Part model, mm, in its own coordinate system. A direction names the side the tool comes from. Round coordinates to 2 decimals unless told otherwise and drop trailing zeros. Use a Markdown table: item, result. Add a question column.
Item 1: Which spindle directions (+Z, -Z, +X, -X, +Y, -Y) get a long thin tool onto all of the face, cutting with end or side? Do faces 1 (the face through (-24.724, 24.297, 1.504)), 2 (the face through (1.1, 27.994, 1.504)), 3 (the face through (1.1, 27.994, 8.496)). Say none if no direction does.
Item 2: Flat gauge pins, fed straight in: pin 1 (12 mm diameter, centred on x = -22.5, y = 18.5, fed in from +Z); pin 2 (1.5 mm diameter, centred on x = -11, z = 1.5, fed in from +Y); pin 3 (1 mm diameter, centred on x = -5.5, z = 9, fed in from -Y); pin 4 (5 mm diameter, centred on x = 0.5, y = 28, fed in from -Z). Where does each tip first touch, or does it go through?
Item 3: Probe line 1 (Y direction, x = -24.5, z = 5); line 2 (X direction, y = 28.25, z = 4.75); line 3 (X direction, y = 31.75, z = 3). List the from-to ranges inside material, lowest first. Write a range as [from, to].
```python
from build123d import *

# Parameters (mm, degrees)
F0_W     = 12
F0_H     = 12
F0_W_2   = 10
F0_H_2   = 10
F1_DEPTH = 10
F2_R     = 4.99999


# Not quite as in the source:
# - a fillet or chamfer is up to 0.001 mm smaller than in the source, because OpenCascade refuses the exact size


with BuildPart() as f1:
    # F0 (on Top) → F1 (new body)
    with BuildSketch(Plane.XY):
        Polygon((2.5256457627, 38.7224316552), (-22.4743542373, 38.7224316552), (-22.4743542373, 25.7224316552), (-22.4743542373, 13.7224316552), (2.5256457627, 13.7224316552), (2.5256457627, 23.7224316552), align=None)
        with Locations((-28.4743542373, 19.7224316552)):
            Rectangle(F0_W, F0_H)
        with Locations((7.5256457627, 18.7224316552)):
            Rectangle(F0_W_2, F0_H_2)
    extrude(amount=F1_DEPTH)

    # F2 (radius 5 in the source; OpenCascade refuses exactly that, so slightly less here)
    f2_edges = [f1.edges().sort_by_distance(p)[0] for p in [
        (-22.474354, 38.722432, 5),
        (-22.474354, 32.222432, 10),
        (-34.474354, 19.722432, 10),
        (-34.474354, 25.722432, 5),
        (-34.474354, 13.722432, 5),
        (-34.474354, 19.722432, 0),
        (2.525646, 31.222432, 10),
        (-9.974354, 38.722432, 10),
        (-28.474354, 25.722432, 10),
        (-10.974354, 13.722432, 10),
        (12.525646, 18.722432, 10),
        (7.525646, 23.722432, 10),
        (2.525646, 38.722432, 5),
        (-9.974354, 38.722432, 0),
        (7.525646, 23.722432, 0),
        (2.525646, 31.222432, 0),
        (-22.474354, 32.222432, 0),
        (-28.474354, 25.722432, 0),
        (-10.974354, 13.722432, 0),
        (12.525646, 18.722432, 0),
        (12.525646, 13.722432, 5),
        (12.525646, 23.722432, 5),
    ]]
    fillet(f2_edges, radius=F2_R)


solid = f1.part
```
A:
| question | item | result |
|---|---|---|
| 1 | face 1 | -Z, -X, +Y |
| 1 | face 2 | -Z, +X, +Y |
| 1 | face 3 | +Z, +X, +Y |
| 2 | pin 1 | stops at z = 10 |
| 2 | pin 2 | stops at y = 37.9 |
| 2 | pin 3 | stops at y = 15.15 |
| 2 | pin 4 | stops at z = 0.02 |
| 3 | line 1 | y = [13.72, 25.72] |
| 3 | line 2 | x = [-22.47, 2.52] |
| 3 | line 3 | x = [-22.06, 2.11] |
